The drawing under review shows one solid part. Ordinate dimensions are in mm from its lowest x, y, z. A direction names the side the tool comes from. Coordinates: 2 decimals unless noted, no trailing zeros. Order: outer loops, then holes, each group sorted by start corner. A loop starts at its lowest first (then second) coordinate and runs counter-clockwise, first axis right, second up. Notation, with made-up numbers: (79.5, 22.5) -> (138.5, 22.5) arc R18 cw to (138.5, 26.5) -> close; hole circle Ø11 at (-16, 83.5). An arc over 180 degrees is marked (long way). Use a Markdown table: item, result. Add a question column.
Q1. Add section A-A (y = 11.68). State the section outline as (x, z) points.
Q2. The part is to be moulded in two halves that separate along Y. For the marked faces 1, 2, 3 and 4, say which applies: pulls with the +Y half, pulls with the -Y half, needs draft (parallel to the pull), parting line crosses it, or undercut.
Q3. Add section D-D (z = 8). State the section outline as (x, y) points, then the cut area to 3 significant figures.
Q4. Insertion check: pin 1 (4.5 mm diameter, centred on x = 9, z = 11.5, fed in from -Y); pin 2 (6.5 mm diameter, centred on y = 11.68, z = 4.79, fed in from -X); pin 3 (2.5 mm diameter, centred on x = 3, y = 3.5, fed in from -Z); pin 4 (4 mm diameter, centred on x = 9.5, y = 6, fed in from -Z). Each pin has a flat end and moves straight along its axis. Give the tip position at first contact, or say it passes through.
Q5. Machinability: for the marked faces 5, 6 and 7, which of the approach directions +Z, -Z, +X, -X, +Y, -Y give a long, thin tool a straight path to every point of the face, cutting with its end or side? Answer none if there is none.
Q6. Add section C-C (x = 5.5). State the section outline as (y, z) points, then the cut area to 3 significant figures.
Q7. Add section B-B (z = 4.79). State the section outline as (x, y) points, then the cut area to 3 significant figures.
Q8. Wall thickness on probe 1 along Y at (x, z) = (5.45, 4.79); probe 2 along Y at (x, z) = (0.5, 11.75); probe 3 along X at (y, z) = (5.25, 6): over which ranges is each line inside the solid? List them lowest first.
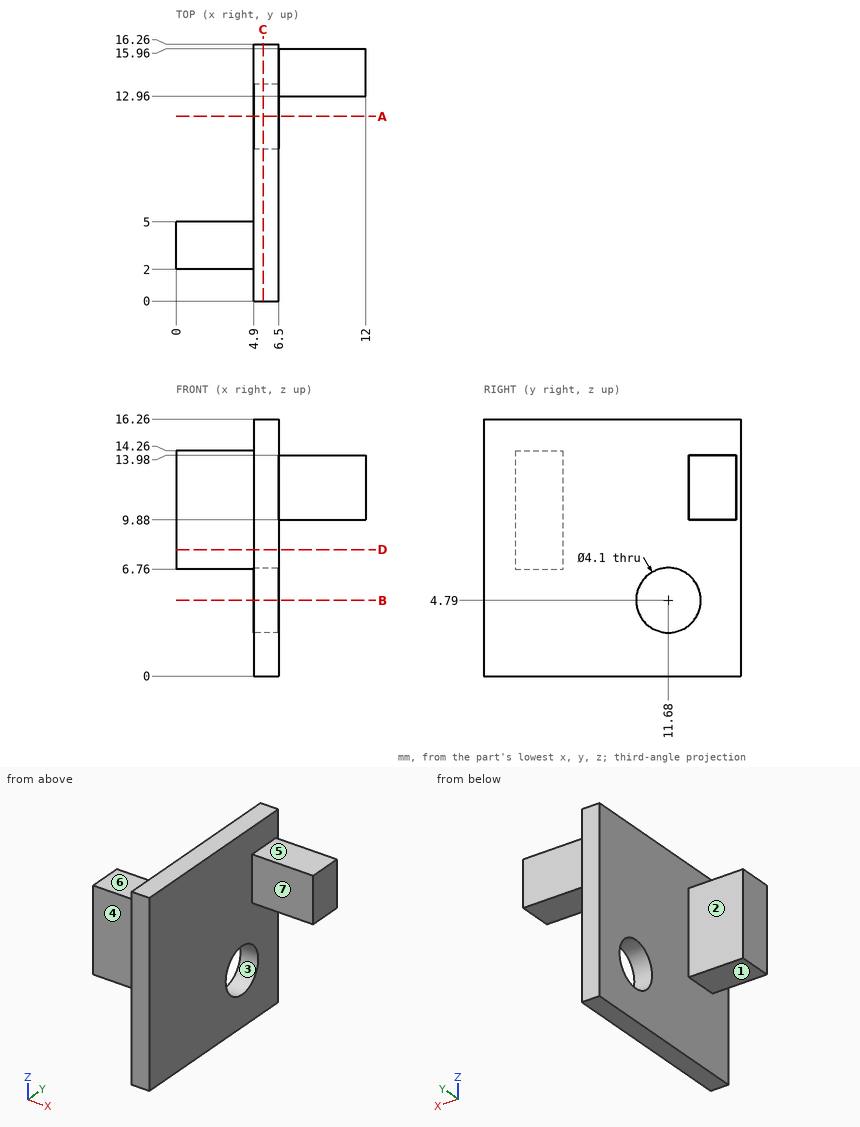
Established:
| question | item | result |
|---|---|---|
| 1 | outline | (4.9, 0) -> (6.5, 0) -> (6.5, 2.74) -> (4.9, 2.74) -> close; (4.9, 6.84) -> (6.5, 6.84) -> (6.5, 16.26) -> (4.9, 16.26) -> close |
| 2 | face 1 | needs draft |
| 2 | face 2 | pulls with the +Y half |
| 2 | face 3 | undercut |
| 2 | face 4 | pulls with the -Y half |
| 3 | outline | (0, 2) -> (4.9, 2) -> (4.9, 0) -> (6.5, 0) -> (6.5, 16.26) -> (4.9, 16.26) -> (4.9, 5) -> (0, 5) -> close |
| 3 | area | 40.7 mm^2 |
| 4 | pin 1 | y = 12.96 |
| 4 | pin 2 | x = 4.9 |
| 4 | pin 3 | z = 6.76 |
| 4 | pin 4 | through |
| 5 | face 5 | +Z, +X, +Y, -Y |
| 5 | face 6 | +Z, -X, +Y, -Y |
| 5 | face 7 | +Z, -Z, +X, -Y |
| 6 | outline | (0, 0) -> (16.26, 0) -> (16.26, 16.26) -> (0, 16.26) -> close; hole circle Ø4.1 at (11.68, 4.79) |
| 6 | area | 251 mm^2 |
| 7 | outline | (4.9, 0) -> (6.5, 0) -> (6.5, 9.63) -> (4.9, 9.63) -> close; (4.9, 13.73) -> (6.5, 13.73) -> (6.5, 16.26) -> (4.9, 16.26) -> close |
| 7 | area | 19.5 mm^2 |
| 8 | probe 1 | 0 to 9.63, 13.73 to 16.26 |
| 8 | probe 2 | 2 to 5 |
| 8 | probe 3 | 4.9 to 6.5 |
